Print and shaded views of the part. All mm, measured from the part's lowest x, y and z. A direction names the side the tool comes from. Round coordinates to 2 decimals unless told otherwise and drop trailing zeros. Write each loop counter-clockwise with the first axis right and the second up, starting at its lowest first coordinate (ties: lowest second). Pieces come first, ordered by that corner, then holes.
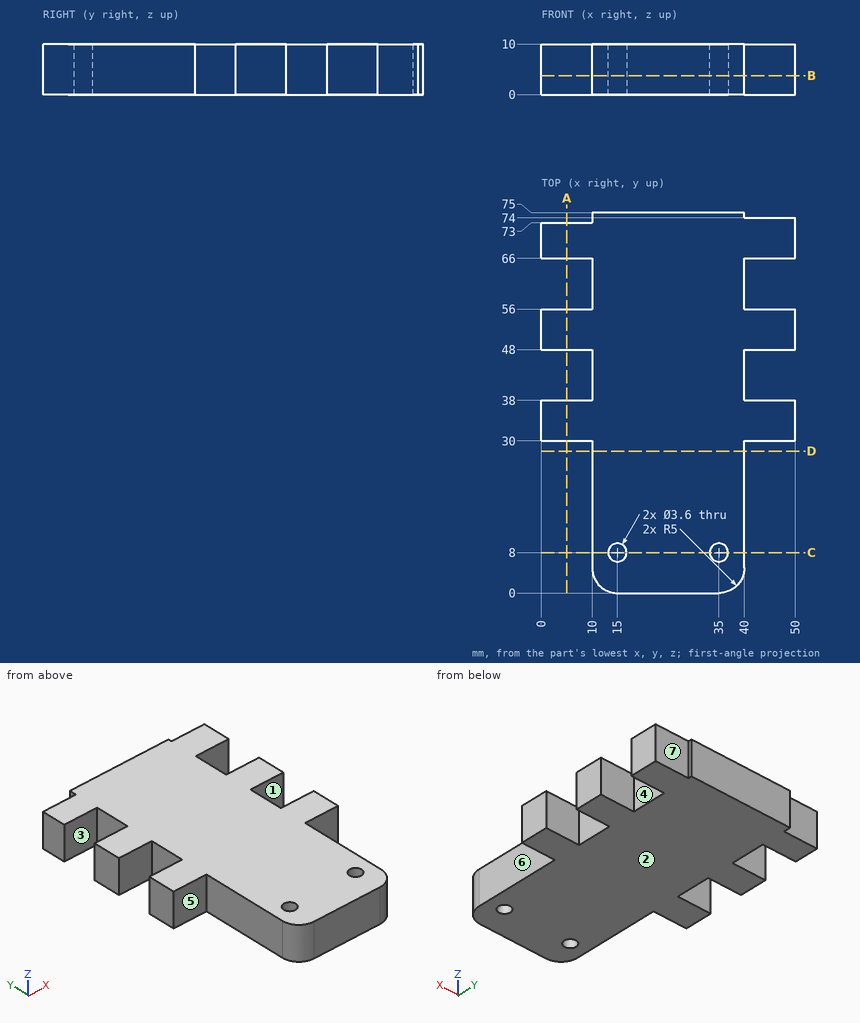
1) Which spindle directions (+Z, -Z, +X, -X, +Y, -Y) get a long thin tool onto all of the face, cutting with end or side? Do the marked faces 1, 2 and 3. Say none if no direction does.
Results:
face 1: +Z, -Z, +X
face 2: -Z, +X, -X, +Y, -Y
face 3: +Z, -Z, -X
2) Slice it at C-C (y = 8). Write the cut outline in (x, z), plus the area to 3 significant figures.
Results:
outline: (10, 0) - (13.2, 0) - (13.2, 10) - (10, 10) - close; (16.8, 0) - (33.2, 0) - (33.2, 10) - (16.8, 10) - close; (36.8, 0) - (40, 0) - (40, 10) - (36.8, 10) - close
area: 228 mm2
3) Slice it at B-B (z = 3.75). Count the separate pieces of the cut face and the enclosed holes in it, plus the area to 3 significant figures.
Results:
separate pieces: 1
enclosed holes: 2
area: 2,690 mm2
4) Slice it at A-A (x = 5). Write the cut outline in (y, z), plus the area to 3 significant figures.
Results:
outline: (30, 0) - (38, 0) - (38, 10) - (30, 10) - close; (48, 0) - (56, 0) - (56, 10) - (48, 10) - close; (66, 0) - (73, 0) - (73, 10) - (66, 10) - close
area: 230 mm2
5) Slice it at D-D (y = 28). Write the cut outline in (x, z), plus the area to 3 significant figures.
Results:
outline: (10, 0) - (40, 0) - (40, 10) - (10, 10) - close
area: 300 mm2
6) Mould opens along Y. For the marked faces 4, 5, 6 and 7 say: released by +Y, released by -Y, zero draft, split by the parting line, or undercut.
Results:
face 4: undercut
face 5: released by -Y
face 6: zero draft
face 7: released by +Y
7) Pin check, flat tips, straight feed: pin 1 Ø3 at (x, y) = (35, 8) entering from -Z; pin 2 Ø3 at (y, z) = (61.5, 7) entering from -X; pin 3 Ø4 at (x, z) = (43.5, 8.5) entering from -Y; pin 4 Ø0.8 at (y, z) = (74.5, 3.5) entering from +X. Stop position of each tip, or through.
Results:
pin 1: passes through
pin 2: stops at x = 10
pin 3: stops at y = 30
pin 4: stops at x = 40
8) Wall check: L1, parallel to Y at x = 8, z = 1; L2, parallel to Y at x = 35, z = 7.25; L3, parallel to X at y = 13, z = 9.5. Give the ranges that are in metal, low to high.
Results:
L1: y = 30 to 38, 48 to 56, 66 to 73
L2: y = 0 to 6.2, 9.8 to 75
L3: x = 10 to 40
